from build123d import *

# Parameters (mm, degrees)
SKETCH1_R           = 1.5
BOSS_EXTRUDE1_DEPTH = 3.125
FILLET1_R           = 10
FILLET2_R           = 15
FILLET3_R           = 30
FILLET4_R           = 30
FILLET5_R           = 80
FILLET6_R           = 30
FILLET7_R           = 5


with BuildPart() as part:
    # Sketch1 → Boss-Extrude1 (new body)
    with BuildSketch(Plane(origin=(0, 0, 0), x_dir=(0, 0, -1), z_dir=(1, 0, 0))):
        Polygon((-143.20422433, -1.13137085), (-143.20422433, -26.13137085), (-64.062088707, -26.13137085), (-52.930717857, -15), (19.6, -15), (19.6, 49.830569927), (-31.940768363, 49.830569927), (-82.90270914, -1.13137085), align=None)
        with Locations((-46.799347007, 3.010764774)):
            Circle(SKETCH1_R, mode=Mode.SUBTRACT)
        with Locations((-14.979541854, 34.830569927)):
            Circle(SKETCH1_R, mode=Mode.SUBTRACT)
        with Locations((-73.810826048, -0.524769132)):
            Circle(SKETCH1_R, mode=Mode.SUBTRACT)
        with Locations((-73.20422433, -16.13137085)):
            Circle(SKETCH1_R, mode=Mode.SUBTRACT)
        with Locations((-133.20422433, -16.13137085)):
            Circle(SKETCH1_R, mode=Mode.SUBTRACT)
        with BuildLine():
            Line((-4.6, 0.75), (-1.854049622, 0.75))
            ThreePointArc((-1.854049622, 0.75), (0, 2), (1.854049622, 0.75))
            Line((1.854049622, 0.75), (4.6, 0.75))
            ThreePointArc((4.6, 0.75), (5.35, 0), (4.6, -0.75))
            Line((4.6, -0.75), (1.854049622, -0.75))
            ThreePointArc((1.854049622, -0.75), (0, -2), (-1.854049622, -0.75))
            Line((-1.854049622, -0.75), (-4.6, -0.75))
            ThreePointArc((-4.6, -0.75), (-5.35, 0), (-4.6, 0.75))
        make_face(mode=Mode.SUBTRACT)
        Polygon((-35.667976157, 0), (-10.83740623, 24.830569927), (-0.4, 24.830569927), (-0.4, 13.742135624), (-14.142135624, 0), align=None, mode=Mode.SUBTRACT)
    extrude(amount=BOSS_EXTRUDE1_DEPTH)

    # Fillet1
    fillet1_edges = [part.edges().sort_by_distance(p)[0] for p in [
        (1.5625, -26.13137085, 143.20422433),
        (1.5625, -1.13137085, 143.20422433),
    ]]
    fillet(fillet1_edges, radius=FILLET1_R)

    # Fillet2
    fillet2_edges = [part.edges().sort_by_distance(p)[0] for p in [
        (1.5625, -15, 52.930717857),
        (1.5625, -26.13137085, 64.062088707),
    ]]
    fillet(fillet2_edges, radius=FILLET2_R)

    # Fillet3
    fillet3_edges = [part.edges().sort_by_distance(p)[0] for p in [
        (1.5625, -15, -19.6),
    ]]
    fillet(fillet3_edges, radius=FILLET3_R)

    # Fillet4
    fillet4_edges = [part.edges().sort_by_distance(p)[0] for p in [
        (1.5625, 49.830569927, 31.940768363),
    ]]
    fillet(fillet4_edges, radius=FILLET4_R)

    # Fillet5
    fillet5_edges = [part.edges().sort_by_distance(p)[0] for p in [
        (1.5625, -1.13137085, 82.90270914),
    ]]
    fillet(fillet5_edges, radius=FILLET5_R)

    # Fillet6
    fillet6_edges = [part.edges().sort_by_distance(p)[0] for p in [
        (1.5625, 49.830569927, -19.6),
    ]]
    fillet(fillet6_edges, radius=FILLET6_R)

    # Fillet7
    fillet7_edges = [part.edges().sort_by_distance(p)[0] for p in [
        (1.5625, 13.742135624, 0.4),
        (1.5625, 24.830569927, 0.4),
        (1.5625, 24.830569927, 10.83740623),
        (1.5625, 0, 35.667976157),
        (1.5625, 0, 14.142135624),
    ]]
    fillet(fillet7_edges, radius=FILLET7_R)


solid = part.part
Input: part model. Units: mm. Frame: model coordinates. A direction names the side the tool comes from. Round coordinates to 2 decimals unless told otherwise and drop trailing zeros. Write each loop counter-clockwise with the first axis right and the second up, starting at its lowest first coordinate (ties: lowest second). Pieces come first, ordered by that corner, then holes.
1) Reachability of faces 4 (the flat face through (2, -0.75, -3)), 5 (the cylindrical face through (1.584, -23.124, 140.353)) from +Z, -Z, +X, -X, +Y, -Y: full face, straight path, thin tool, end or side. Return the list, or none.
2) Cut plane B-B (x = 2.4). Count the separate pieces of the cut face and the enclosed holes in it, then the cut area to 3 significant figures.
3) Cut plane A-A (z = 119). Return the cut outline in (x, y) (3 decimals), then the cut area to 3 significant figures.
4) Cut plane C-C (z = 37.5). Return the cut outline in (x, y) (3 decimals), then the cut area to 3 significant figures.
5) Draft query along Y for faces 1 (the cylindrical face through (1.6, 23.3, 1.8)), 2 (the cylindrical face through (1.58, 47.61, 30.84)), 3 (the flat face through (3.125, 4, 45)). Return one class per face: pulls with the +Y half, pulls with the -Y half, needs draft (parallel to the pull), parting line crosses it, or undercut.
6) Ray query, L1, parallel to Z at x = 2.1, y = 19; L2, parallel to Z at x = 2.9, y = 13.5; L3, parallel to Y at x = 0.5, z = 72.5. Return the intervals inside material, ascending.
7) Contact query for flat-ended pins moving along their axis: P1, Ø2.5, axis at y = 34.83, z = 14.98, coming from the +X side; P2, Ø1.6, axis at x = 1, z = 124.5, coming from the +Y side; P3, Ø3.5, axis at y = -0.52, z = 73.81, coming from the +X side (3 decimals); P4, Ø0.8, axis at x = 2, z = -3, coming from the -Y side. Output: stop coordinate, or through.
Geometry says:
1. face 4: +X, -X
1. face 5: +Z, +X, -X, -Y
2. separate pieces: 1
2. enclosed holes: 7
2. area: 6,320 mm2
3. outline: (0, -26.131) - (3.125, -26.131) - (3.125, -1.131) - (0, -1.131) - close
3. area: 78.1 mm2
4. outline: (0, -15) - (3.125, -15) - (3.125, 43.841) - (0, 43.841) - close
4. area: 184 mm2
5. face 1: undercut
5. face 2: pulls with the +Y half
5. face 3: needs draft
6. L1: z = -19.6 to 0.4, 16.67 to 62.98
6. L2: z = -19.56 to 0.97, 22.17 to 69.92
6. L3: y = -26.13 to -17.46, -14.81 to -1.25, 0.2 to 11.75
7. P1: passes through
7. P2: stops at y = -1.13
7. P3: stops at x = 3.125
7. P4: stops at y = -12.04
